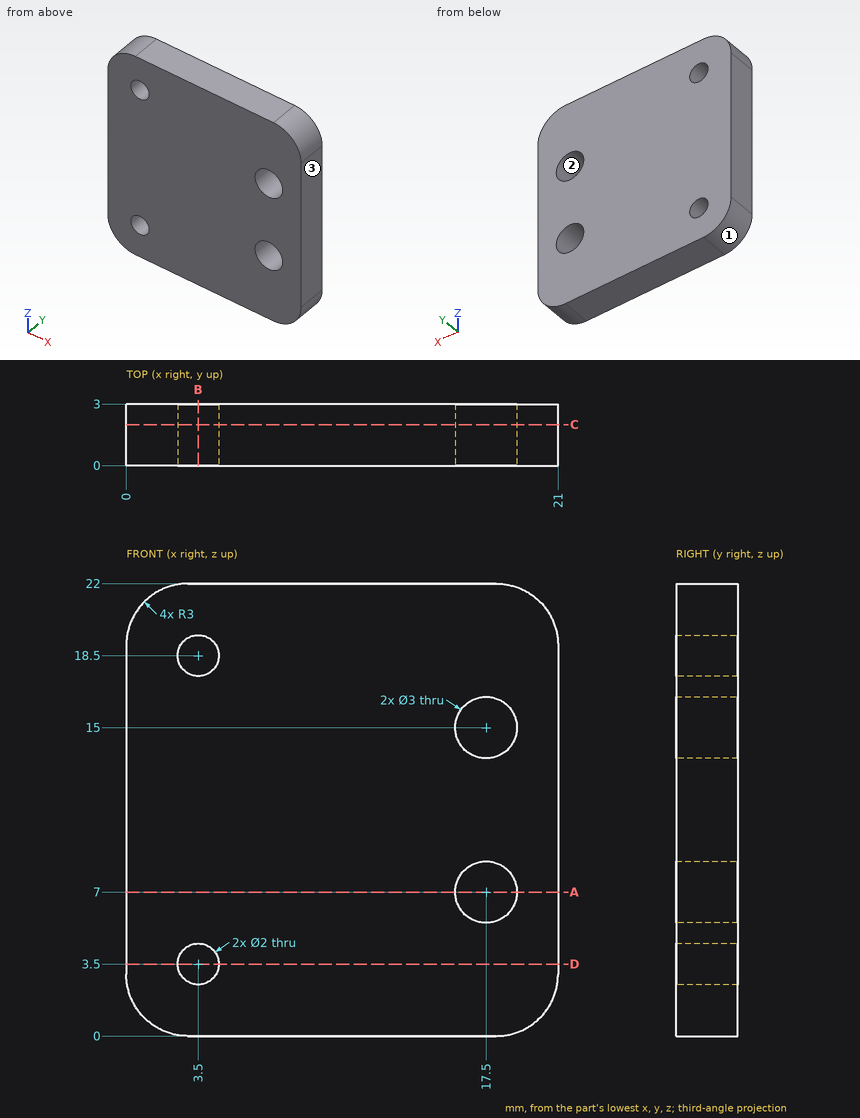
Geometry check sheet. Reference: drawing and pictorial views, mm from the part's lowest x, y, z. Round coordinates to 2 decimals unless told otherwise and drop trailing zeros. Order: outer loops, then holes, each group sorted by start corner. A loop starts at its lowest first (then second) coordinate and runs counter-clockwise, first axis right, second up. Notation, with made-up numbers: (87.25, 6) - (104.25, 6) arc R22 cw to (104.25, 41) - close; hole circle Ø2 at (38.25, -33.75). An arc over 180 degrees is marked (long way). Use a Markdown table: item, result. Add a question column.
1) Gauge pin test, flat end, axial feed: P1, Ø2.5, axis at x = 17.5, z = 15, coming from the -Y side. Record the tip position at first contact, or that the pin passes through.
2) Section check B-B (x = 3.5). Record the cut outline in (y, z).
3) Section check C-C (y = 2). Record the cut outline in (x, z), then the cut area to 3 significant figures.
4) Section check D-D (z = 3.5). Record the cut outline in (x, y).
5) Thickness scan on line 1 along X through (y, z) = (2.35, 15); line 2 along X through (y, z) = (2.2, 18.5); line 3 along Z through (x, y) = (18, 0.95). Record the ranges inside material, lowest first.
6) Section check A-A (z = 7). Record the cut outline in (x, y).
7) Mould release check, pull along X, two halves, no side actions. Record for the marked faces 1, 2 and 3: released by +X, released by -X, zero draft, split by the parting line, or undercut.
Established:
| question | item | result |
|---|---|---|
| 1 | P1 | through |
| 2 | outline | (0, 0) - (3, 0) - (3, 2.5) - (0, 2.5) - close; (0, 4.5) - (3, 4.5) - (3, 17.5) - (0, 17.5) - close; (0, 19.5) - (3, 19.5) - (3, 22) - (0, 22) - close |
| 3 | outline | (0, 3) arc R3 ccw to (3, 0) - (18, 0) arc R3 ccw to (21, 3) - (21, 19) arc R3 ccw to (18, 22) - (3, 22) arc R3 ccw to (0, 19) - close; hole circle Ø2 at (3.5, 3.5); hole circle Ø2 at (3.5, 18.5); hole circle Ø3 at (17.5, 7); hole circle Ø3 at (17.5, 15) |
| 3 | area | 434 mm2 |
| 4 | outline | (0, 0) - (2.5, 0) - (2.5, 3) - (0, 3) - close; (4.5, 0) - (21, 0) - (21, 3) - (4.5, 3) - close |
| 5 | line 1 | 0 to 16, 19 to 21 |
| 5 | line 2 | 0 to 2.5, 4.5 to 21 |
| 5 | line 3 | 0 to 5.59, 8.41 to 13.59, 16.41 to 22 |
| 6 | outline | (0, 0) - (16, 0) - (16, 3) - (0, 3) - close; (19, 0) - (21, 0) - (21, 3) - (19, 3) - close |
| 7 | face 1 | released by -X |
| 7 | face 2 | undercut |
| 7 | face 3 | released by +X |
